from build123d import *

# Parameters (mm, degrees)
F0_W          = 15
F0_H          = 130
F2_R          = 5
F3_DEPTH      = 93.5532969241
F3_DEPTH_BACK = 25
F4_R          = 11
F5_DEPTH      = 3.5


with BuildPart() as f1:
    # F0 (on Front) → F1 (revolve)
    with BuildSketch(Plane.XZ):
        with Locations((-7.6752220338, -28.5522969241)):
            Rectangle(F0_W, F0_H)
    revolve(axis=Axis((-0.1752220338, 0, -28.5522969241), (0, 0, -1)))

    # F2 (on Top) → F3 (cut, two sides)
    with BuildSketch(Plane.XY) as f3_sk:
        Circle(F2_R)
    extrude(amount=-F3_DEPTH, mode=Mode.SUBTRACT)
    extrude(f3_sk.sketch, amount=F3_DEPTH_BACK, mode=Mode.SUBTRACT)

    # F4 (on face) → F5 (cut)
    with BuildSketch(Plane(origin=(0, 0, -93.5522969241), x_dir=(1, 0, 0), z_dir=(0, 0, -1))):
        with Locations((-0.1752220338, 0)):
            Circle(F4_R)
    extrude(amount=-F5_DEPTH, mode=Mode.SUBTRACT)


solid = f1.part
The model under review builds one solid part; all positions refer to its coordinate system, in mm. A direction names the side the tool comes from. Coordinates: 2 decimals unless noted, no trailing zeros. Loops run counter-clockwise (first coordinate to the right, second up) from the corner with the lowest first, then second, coordinate; pieces in that order, holes last. Notation, with made-up numbers: (-25.5, -2) -> (-20.5, -2) arc R12 ccw to (-20.5, 15) -> close; hole circle Ø6 at (-31.75, -36.75). An arc over 180 degrees is marked (long way). Use a Markdown table: item, result. Add a question column.
1. Machinability: for faces 4 (the face through (0, 0, 25)), 5 (the face through (8, 8, -93.552)), which of the approach directions +Z, -Z, +X, -X, +Y, -Y give a long, thin tool a straight path to every point of the face, cutting with its end or side? Answer none if there is none.
2. To check wall thickness, follow line 1 (Y direction, x = 0, z = -22.5); line 2 (Z direction, x = 6, y = -2); line 3 (X direction, y = -2.25, z = -34). State the ranges of each line that lie inside material, in increasing order.
3. Add section A-A on y = 0. Write out the cut boundary in (x, z), plus the area to 3 significant figures.
4. Add section C-C on z = -2. Write out the cut boundary in (x, y), plus the area to 3 significant figures.
5. Draft analysis for pull direction Y (two halves, no side actions). For faces 1 (the face through (-14.48, 4.51, -27.64)), 2 (the face through (0, 0, 36.448)), 3 (the face through (-2.56, 10.74, -91.83)), state which applies: pulls with the +Y half, pulls with the -Y half, needs draft (parallel to the pull), parting line crosses it, or undercut.
6. Add section D-D on x = -8.5. Write out the cut boundary in (y, z).
7. Add section B-B on x = -2.5. Write out the cut boundary in (y, z), plus the area to 3 significant figures.
8. Clearance check with flat-ended pins moving along their axes: pin 1 Ø5 at (x, z) = (10.5, -15.5) entering from -Y; pin 2 Ø6 at (x, y) = (0, 0) entering from -Z; pin 3 Ø3 at (y, z) = (9.5, 13.5) entering from +X. State where each tip first meets the part, or that it passes through.
Returned:
| question | item | result |
|---|---|---|
| 1 | face 4 | -Z |
| 1 | face 5 | -Z, +X, -X, +Y, -Y |
| 2 | line 1 | y = -15 to -5, 5 to 15 |
| 2 | line 2 | z = -90.05 to 36.45 |
| 2 | line 3 | x = -15.01 to -4.47, 4.47 to 14.66 |
| 3 | outline | (-15.18, -93.55) -> (-11.18, -93.55) -> (-11.18, -90.05) -> (-5, -90.05) -> (-5, 25) -> (5, 25) -> (5, -90.05) -> (10.82, -90.05) -> (10.82, -93.55) -> (14.82, -93.55) -> (14.82, 36.45) -> (-15.18, 36.45) -> close |
| 3 | area | 2,670 mm² |
| 4 | outline | circle Ø30 at (-0.18, 0); hole circle Ø10 at (0, 0) |
| 4 | area | 628 mm² |
| 5 | face 1 | parting line crosses it |
| 5 | face 2 | needs draft |
| 5 | face 3 | undercut |
| 6 | outline | (-12.48, -93.55) -> (-7.19, -93.55) -> (-7.19, -90.05) -> (7.19, -90.05) -> (7.19, -93.55) -> (12.48, -93.55) -> (12.48, 36.45) -> (-12.48, 36.45) -> close |
| 7 | outline | (-14.82, -93.55) -> (-10.75, -93.55) -> (-10.75, -90.05) -> (-4.33, -90.05) -> (-4.33, 25) -> (4.33, 25) -> (4.33, -90.05) -> (10.75, -90.05) -> (10.75, -93.55) -> (14.82, -93.55) -> (14.82, 36.45) -> (-14.82, 36.45) -> close |
| 7 | area | 2,780 mm² |
| 8 | pin 1 | stops at y = -12.58 |
| 8 | pin 2 | stops at z = 25 |
| 8 | pin 3 | stops at x = 12.51 |
